from build123d import *

# Parameters (mm, degrees)
F0_R     = 52.5
F1_DEPTH = 84
F2_T     = -5
F3_R     = 47.5
F3_R_2   = 45.5
F4_DEPTH = 62
F5_R     = 3
F7_DEPTH = 3


with BuildPart() as f1:
    # F0 (on Top) → F1 (new body)
    with BuildSketch(Plane.XY):
        Circle(F0_R)
    extrude(amount=F1_DEPTH)

    # F2
    f2_openings = [f1.faces().sort_by_distance(p)[0] for p in [
        (0, 0, 84),
    ]]
    offset(amount=F2_T, openings=f2_openings)

    # F3 (on face) → F4 (join)
    with BuildSketch(Plane.XY.offset(5)):
        Circle(F3_R)
        Circle(F3_R_2, mode=Mode.SUBTRACT)
    extrude(amount=F4_DEPTH)

    # F5
    f5_edges = [f1.edges().sort_by_distance(p)[0] for p in [
        (-52.5, 0, 0),
    ]]
    fillet(f5_edges, radius=F5_R)

    # F6 (on face) → F7 (join)
    with BuildSketch(Plane.XY.offset(67)):
        with BuildLine():
            ThreePointArc((5.2092810259, 47.2134873865), (2.6085771162, 47.4283177588), (0, 47.5))
            Line((0, 47.5), (0, 45.5))
            ThreePointArc((0, 45.5), (2.4987422903, 45.4313359584), (4.9899428775, 45.2255510755))
            Line((4.9899428775, 45.2255510755), (5.2092810259, 47.2134873865))
        make_face()
    extrude(amount=F7_DEPTH)


solid = f1.part
Can you work these out from the model? Positions are in its coordinate system, mm. A direction names the side the tool comes from. Give positions to 0.01 mm unless a question says otherwise; leave off trailing zeros. Write each loop counter-clockwise with the first axis right and the second up, starting at its lowest first coordinate (ties: lowest second). Pieces come first, ordered by that corner, then holes. Notation, with made-up numbers: M 67.5,-33 L 99.5,-33 A5 cw 99.5,-28 Z; hole C -34,35 d3. An arc over 180 degrees is marked long. Answer in a Markdown table with one row per item. Add a question column.
Item 1: Imagine slicing it at B-B, the plane z = 35.5. Write out the boundary of the cut face in (x, y), plus the area to 3 significant figures.
Item 2: Please list where these lines run through material, in increasing order: L1, parallel to Y at x = 0, z = 45; L2, parallel to Z at x = 21.5, y = 6.
Item 3: Imagine slicing it at A-A, the plane y = 0. Write out the boundary of the cut face in (x, z), plus the area to 3 significant figures.
Item 4: We'd pull the mould along X, two halves only. Please class faces 1 (the flat face through (-1, 1, 5)), 2 (the flat face through (-1, 1, 0)), 3 (the cylindrical face through (50.076, 15.77, 42.933)): released by +X, released by -X, zero draft, split by the parting line, or undercut.
Item 5: On a 3-axis mill with a long thin cutter (end or side, diameter ignored), from which of +Z, -Z, +X, -X, +Y, -Y can I reach the whole of each face in a straight line? I mean faces 4 (the flat face through (0, -46, 67)), 5 (the flat face through (-11.9, -46.4, 84)). Say none if no direction works.
Item 6: For pin 1 Ø1.6 at (y, z) = (47, 68.5) entering from -X; pin 2 Ø1 at (y, z) = (10.5, 27.5) entering from -X; pin 3 Ø3 at (x, y) = (-24, 12.5) entering from +Z, each with a flat end and sliding along its axis, tell me the tip position at first contact or that it passes through.
Evaluation:
| question | item | result |
|---|---|---|
| 1 | outline | C 0,0 d105; hole C 0,0 d91 |
| 1 | area | 2,160 mm² |
| 2 | L1 | y = -52.5 to -45.5, 45.5 to 52.5 |
| 2 | L2 | z = 0 to 5 |
| 3 | outline | M -52.5,3 A3 ccw -49.5,0 L 49.5,0 A3 ccw 52.5,3 L 52.5,84 L 47.5,84 L 47.5,67 L 45.5,67 L 45.5,5 L -45.5,5 L -45.5,67 L -47.5,67 L -47.5,84 L -52.5,84 Z |
| 3 | area | 1,560 mm² |
| 4 | face 1 | undercut |
| 4 | face 2 | zero draft |
| 4 | face 3 | split by the parting line |
| 5 | face 4 | +Z |
| 5 | face 5 | +Z, +X, -X, +Y, -Y |
| 6 | pin 1 | stops at x = -24.94 |
| 6 | pin 2 | stops at x = -51.54 |
| 6 | pin 3 | stops at z = 5 |
